```python
from build123d import *

# Parameters (mm, degrees)
BOSS_EXTRU_1_DEPTH             = 4
ENL_V_START                    = -4
ENL_V_MAT_EXTRU_3_DEPTH        = 3.6
CONG_2_R                       = 3
CONG_3_R                       = 3
CONG_2_OF_SYM_TRIE1_R          = 3
CONG_3_OF_SYM_TRIE1_R          = 3
F_4_8_4_8_DIAMETER_HOLE2_D     = 4.8
F_4_8_4_8_DIAMETER_HOLE2_DEPTH = 6.4
F_4_8_4_8_DIAMETER_HOLE2_TIP   = 1.442065486
CHANFREIN1_SIZE                = 0.5
ESQUISSE9_R                    = 4.5
ENL_V_MAT_EXTRU_4_DEPTH        = 1.1
CONG_4_R                       = 1


with BuildPart() as part:
    # Esquisse1 → Révolution1 (revolve)
    with BuildSketch(Plane.XY, mode=Mode.PRIVATE) as r_volution1_sk:
        Polygon((-6.5, -4), (-6.5, -5.5), (-10, -5.5), (-10, 2.1), (-8, 2.1), (-8, 1.1), (-8.4, 1.1), (-8.4, 0), (-8, 0), (-8, -4), align=None)
    revolve(r_volution1_sk.sketch.rotate(Axis((0, 6.608552154, 0), (0, -1, 0)), 270), axis=Axis((0, 6.608552154, 0), (0, -1, 0)))

    # Esquisse2 → Boss.-Extru.1 (add)
    with BuildSketch(Plane(origin=(0, 2.1, 0), x_dir=(1, 0, 0), z_dir=(0, 1, 0))):
        with BuildLine():
            Line((-12.5, -4), (-9.16515139, -4))
            ThreePointArc((-9.16515139, -4), (-10, 0), (-9.16515139, 4))
            Line((-9.16515139, 4), (-12.5, 4))
            ThreePointArc((-12.5, 4), (-16.5, 0), (-12.5, -4))
        make_face()
    boss_extru_1 = extrude(amount=-BOSS_EXTRU_1_DEPTH)

    # Esquisse2<6> → Enlèv. mat.-Extru.3 (cut)
    with BuildSketch(Plane(origin=(0, 2.1, 0), x_dir=(1, 0, 0), z_dir=(0, 1, 0)).offset(ENL_V_START)):
        with BuildLine():
            ThreePointArc((-9.5, 3.122498999), (-10, 0), (-9.5, -3.122498999))
            Line((-9.5, -3.122498999), (-9.5, 3.122498999))
        make_face()
    enl_v_mat_extru_3 = extrude(amount=-ENL_V_MAT_EXTRU_3_DEPTH, mode=Mode.SUBTRACT)

    # Congé2
    cong_2_edges = [part.edges().sort_by_distance(p)[0] for p in [
        (-9.5, -3.7, 3.122498999),
        (-9.5, -3.7, -3.122498999),
    ]]
    fillet(cong_2_edges, radius=CONG_2_R)

    # Congé3
    cong_3_edges = [part.edges().sort_by_distance(p)[0] for p in [
        (-9.16515139, 0.1, -4),
        (-9.16515139, 0.1, 4),
    ]]
    fillet(cong_3_edges, radius=CONG_3_R)

    # Symétrie1: Boss.-Extru.1, Enlèv. mat.-Extru.3 across plane
    add(boss_extru_1.mirror(Plane(origin=(0, 0, 0), x_dir=(0, 0, 1), z_dir=(1, 0, 0))))
    add(enl_v_mat_extru_3.mirror(Plane(origin=(0, 0, 0), x_dir=(0, 0, 1), z_dir=(1, 0, 0))), mode=Mode.SUBTRACT)

    # Congé2 of Symétrie1
    cong_2_of_sym_trie1_edges = [part.edges().sort_by_distance(p)[0] for p in [
        (9.5, -3.7, 3.122498999),
        (9.5, -3.7, -3.122498999),
    ]]
    fillet(cong_2_of_sym_trie1_edges, radius=CONG_2_OF_SYM_TRIE1_R)

    # Congé3 of Symétrie1
    cong_3_of_sym_trie1_edges = [part.edges().sort_by_distance(p)[0] for p in [
        (9.16515139, 0.1, -4),
        (9.16515139, 0.1, 4),
    ]]
    fillet(cong_3_of_sym_trie1_edges, radius=CONG_3_OF_SYM_TRIE1_R)

    # Ø4.8 (4.8) Diameter Hole2
    with Locations(Plane(origin=(0, 2.1, 0), x_dir=(1, 0, 0), z_dir=(0, 1, 0))):
        with Locations((-12.5, 0), (12.5, 0)):
            Hole(F_4_8_4_8_DIAMETER_HOLE2_D / 2, depth=F_4_8_4_8_DIAMETER_HOLE2_DEPTH)
            with Locations((0, 0, -(F_4_8_4_8_DIAMETER_HOLE2_DEPTH + F_4_8_4_8_DIAMETER_HOLE2_TIP / 2))):  # 118° drill point
                Cone(0, F_4_8_4_8_DIAMETER_HOLE2_D / 2, F_4_8_4_8_DIAMETER_HOLE2_TIP, mode=Mode.SUBTRACT)

    # Chanfrein1
    chanfrein1_edges = [part.edges().sort_by_distance(p)[0] for p in [
        (14.9, 2.1, 0),
        (-10.1, 2.1, 0),
    ]]
    chamfer(chanfrein1_edges, length=CHANFREIN1_SIZE)

    # Esquisse9 → Enlèv. mat.-Extru.4 (cut)
    with BuildSketch(Plane.XZ.offset(5.5)):
        with Locations((-12.5, 0)):
            Circle(ESQUISSE9_R)
        with Locations((12.5, 0)):
            Circle(ESQUISSE9_R)
    extrude(amount=-ENL_V_MAT_EXTRU_4_DEPTH, mode=Mode.SUBTRACT)

    # Congé4
    # the kernel refuses this fillet: 1 mm, written as the material it takes off along each edge
    with BuildSketch(Plane(origin=(9.421052632, -4.4, 3.281780477), x_dir=(-0.686560042836171, 0, -0.7270731102033653), z_dir=(0, -1, 0))) as cong_4_piece_1:
        with BuildLine():
            CenterArc((0.604915781, -0.998168708), CONG_4_R, 93.468029374, 62.964308211)
            Line((-0.311672758, -0.598336932), (-0.403331612, -0.558353754))
            ThreePointArc((-0.403331612, -0.558353754), (-0.310284429, -0.351422835), (-0.083419367, 0.05514716))
            Line((-0.083419367, 0.05514716), (0.006049158, 0.099816871))
            ThreePointArc((0.006049158, 0.099816871), (0.272212102, 0.091759185), (0.538375045, 0.099816871))
            Line((0.538375045, 0.099816871), (0.544424203, 0))
        make_face()
    extrude(amount=2.786614567, mode=Mode.SUBTRACT)
    with BuildSketch(Plane(origin=(9.421052632, -4.4, -3.281780477), x_dir=(-0.6865600428361709, 0, 0.7270731102033654), z_dir=(0, -1, 0)), Plane(origin=(-9.421052632, -4.4, 3.281780477), x_dir=(0.6865600428361707, 0, -0.7270731102033658), z_dir=(0, -1, 0))) as cong_4_piece_2:
        with BuildLine():
            CenterArc((0.604915781, 0.998168708), CONG_4_R, 203.567662416, 62.964308211)
            Line((-0.311672758, 0.598336932), (-0.403331612, 0.558353754))
            ThreePointArc((-0.403331612, 0.558353754), (-0.310284429, 0.351422835), (-0.083419367, -0.05514716))
            Line((-0.083419367, -0.05514716), (0.006049158, -0.099816871))
            ThreePointArc((0.006049158, -0.099816871), (0.272212102, -0.091759185), (0.538375045, -0.099816871))
            Line((0.538375045, -0.099816871), (0.544424203, 0))
        make_face()
    extrude(amount=2.786614567, mode=Mode.SUBTRACT)
    with BuildSketch(Plane(origin=(-9.421052632, -4.4, -3.281780477), x_dir=(0.3276573021844398, 0, -0.9447966407249841), z_dir=(0, -1, 0))) as cong_4_piece_3:
        with BuildLine():
            CenterArc((0.605807396, 0.997627822), CONG_4_R, 210.982965052, 62.964308211)
            Line((-0.251512996, 0.482844619), (-0.337245035, 0.431366299))
            ThreePointArc((-0.337245035, 0.431366299), (-0.207136841, 0.199031418), (-0.091321217, -0.04074844))
            Line((-0.091321217, -0.04074844), (-0.010371424, -0.099460714))
            ThreePointArc((-0.010371424, -0.099460714), (0.455018696, -0.112838034), (0.68152967, -0.099762782))
            Line((0.68152967, -0.099762782), (0.674645827, 0))
        make_face()
    extrude(amount=2.786614567, mode=Mode.SUBTRACT)


solid = part.part
```
Can you work these out from the model? Positions are in its coordinate system, mm. A direction names the side the tool comes from. Round coordinates to 2 decimals unless told otherwise and drop trailing zeros. Loops run counter-clockwise (first coordinate to the right, second up) from the corner with the lowest first, then second, coordinate; pieces in that order, holes last.
Item 1: Suppose I cut it at B-B, the plane y = -0.5. Write out the boundary of the cut face in (x, z), then the cut area to 3 significant figures.
Item 2: Suppose I cut it at C-C, the plane z = 0. State how many separate pieces and enclosed holes the cut face has, then the cut area to 3 significant figures.
Item 3: Will these pins go through, and if not, where does the flat tip stop? pin 1 Ø0.8 at (x, z) = (-9, -0.5) entering from -Y; pin 2 Ø4 at (x, z) = (-14, 2.5) entering from -Y; pin 3 Ø0.5 at (x, y) = (12, -0.5) entering from -Z; pin 4 Ø10.5 at (x, z) = (0, 0) entering from +Y.
Item 4: Please list where these lines run through material, in increasing order: L1, parallel to X at y = 0.1, z = 0; L2, parallel to X at y = -1.6, z = 0; L3, parallel to Z at x = -12.5, y = -0.5.
Item 5: Suppose I cut it at A-A, the plane x = 0. Write out the boundary of the cut face in (y, z).
Item 6: Suppose I cut it at D-D, the plane x = -4.5. Write out the boundary of the cut face in (y, z).
Item 7: Which directions (+Z, -Z, +X, -X, +Y, -Y) give clear straight access to the entire face, cutting with the end or side of a thin tool? Please do faces 1 (the flat face through (12, 0, 4)), 2 (the cylindrical face through (-9.444, -3.168, -3.173)), 3 (the flat face through (9, -4.4, 0)).
Reported:
1. outline: (-12.5, -4) - (-10.95, -4) arc R3 cw to (-8.43, -5.38) arc R10 ccw to (8.43, -5.38) arc R3 cw to (10.95, -4) - (12.5, -4) arc R4 ccw to (12.5, 4) - (10.95, 4) arc R3 cw to (8.43, 5.38) arc R10 ccw to (-8.43, 5.38) arc R3 cw to (-10.95, 4) - (-12.5, 4) arc R4 ccw to start; hole circle Ø4.8 at (-12.5, 0); hole circle Ø16 at (0, 0); hole circle Ø4.8 at (12.5, 0)
1. area: 174 mm2
2. separate pieces: 4
2. enclosed holes: 0
2. area: 40.2 mm2
3. pin 1: stops at y = -4.4
3. pin 2: stops at y = -1.9
3. pin 3: stops at z = -4
3. pin 4: passes through
4. L1: x = -16.5 to -14.9, -10.1 to -8.4, 8.4 to 10.1, 14.9 to 16.5
4. L2: x = -16.5 to -14.9, -10.1 to -8, 8 to 10.1, 14.9 to 16.5
4. L3: z = -4 to -2.4, 2.4 to 4
5. outline: (-5.5, -10) - (2.1, -10) - (2.1, -8) - (1.1, -8) - (1.1, -8.4) - (0, -8.4) - (0, -8) - (-4, -8) - (-4, -6.5) - (-5.5, -6.5) - close; (-5.5, 6.5) - (-4, 6.5) - (-4, 8) - (0, 8) - (0, 8.4) - (1.1, 8.4) - (1.1, 8) - (2.1, 8) - (2.1, 10) - (-5.5, 10) - close
6. outline: (-5.5, -8.93) - (2.1, -8.93) - (2.1, -6.61) - (1.1, -6.61) - (1.1, -7.09) - (0, -7.09) - (0, -6.61) - (-4, -6.61) - (-4, -4.69) - (-5.5, -4.69) - close; (-5.5, 4.69) - (-4, 4.69) - (-4, 6.61) - (0, 6.61) - (0, 7.09) - (1.1, 7.09) - (1.1, 6.61) - (2.1, 6.61) - (2.1, 8.93) - (-5.5, 8.93) - close
7. face 1: +Z, +X, +Y, -Y
7. face 2: -Z, -X, -Y
7. face 3: +X, -Y
